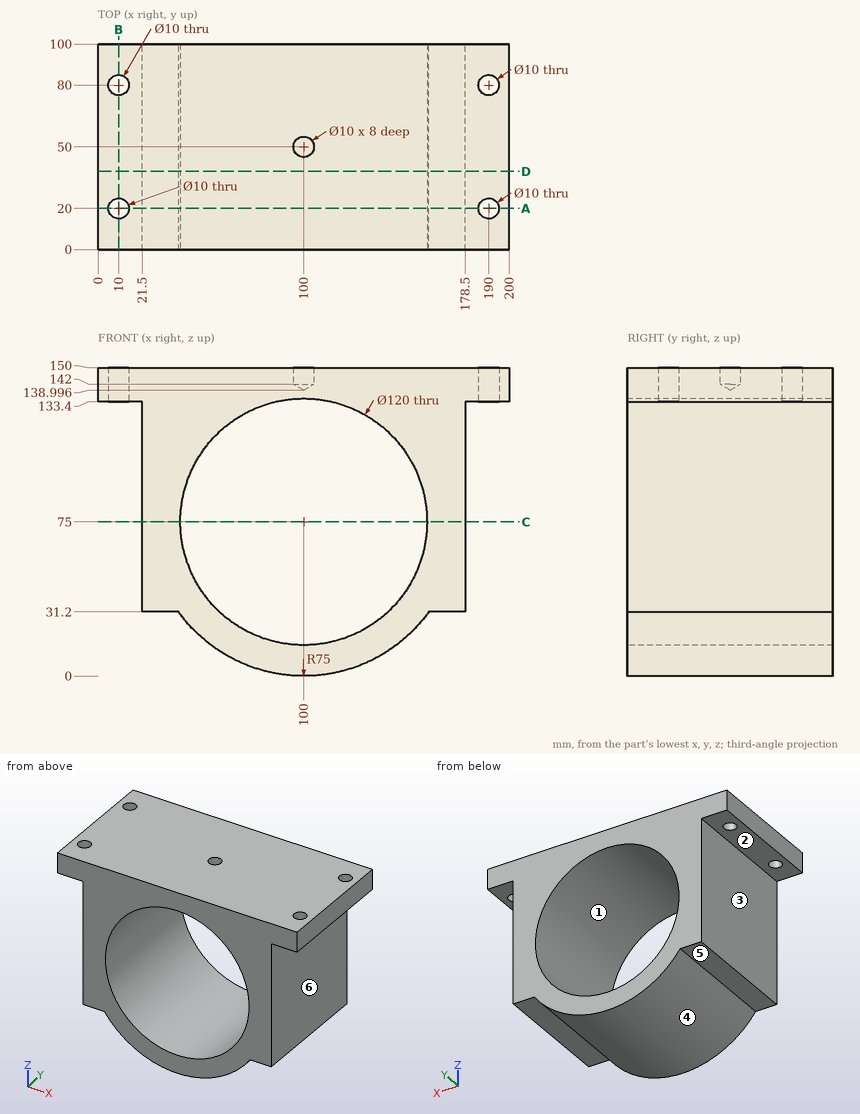
Answer from the drawing. Dimensions are ordinates in mm from the lowest x, y and z of the part. A direction names the side the tool comes from. Give positions to 0.01 mm unless a question says otherwise; leave off trailing zeros. Order: outer loops, then holes, each group sorted by start corner. A loop starts at its lowest first (then second) coordinate and runs counter-clockwise, first axis right, second up. Notation, with made-up numbers: (2.5, 77) - (34.5, 77) arc R22 ccw to (34.5, 100) - close; hole circle Ø10 at (32, 26.5). An arc over 180 degrees is marked (long way). One line per item, written item: value. Start each with the question number.
1) A cutting plane is placed at C-C on z = 75. Give the vertices of the cut face in (x, y), then the cut area to 3 significant figures.
2) A tool of negligible diameter and unlimited length cuts with its end or side. For the marked faces 4, 5 and 6, from which of +Z, -Z, +X, -X, +Y, -Y can it reach the whole face along a straight path? Write none if from no direction.
3) Find the intervals of material crossed by L1, parallel to Y at x = 10, z = 144.5; L2, parallel to Z at x = 98.5, y = 14 (1 decimal); L3, parallel to X at y = 26.5, z = 75, in increasing order.
4) A cutting plane is placed at D-D on y = 38. Give the vertices of the cut face in (x, z).
5) The mould has two halves that part along X. Classify the marked faces 1, 2 and 3: released by +X, released by -X, zero draft, split by the parting line, or undercut.
6) Given pin 1 Ø19.5 at (x, y) = (28.5, 59) entering from -Z; pin 2 Ø8 at (x, y) = (10, 20) entering from -Z; pin 3 Ø16 at (x, y) = (10, 80) entering from -Z; pin 4 Ø3 at (y, z) = (81.5, 27.5) entering from -X, each flat-ended and moving along its own axis, determine where each tip first touches the part or whether it passes through.
7) A cutting plane is placed at A-A on y = 20. Give the vertices of the cut face in (x, z), then the cut area to 3 significant figures.
8) A cutting plane is placed at B-B on x = 10. Give the vertices of the cut face in (y, z).
Answer sheet:
1. outline: (21.5, 0) - (40, 0) - (40, 100) - (21.5, 100) - close; (160, 0) - (178.5, 0) - (178.5, 100) - (160, 100) - close
1. area: 3,700 mm2
2. face 4: -Z, +Y, -Y
2. face 5: -Z, -X, +Y, -Y
2. face 6: -Z, +X, +Y, -Y
3. L1: y = 0 to 15, 25 to 75, 85 to 100
3. L2: z = 0 to 15, 135 to 150
3. L3: x = 21.5 to 40, 160 to 178.5
4. outline: (0, 133.4) - (21.5, 133.4) - (21.5, 31.2) - (39.12, 31.2) arc R75 ccw to (160.88, 31.2) - (178.5, 31.2) - (178.5, 133.4) - (200, 133.4) - (200, 150) - (0, 150) - close; hole circle Ø120 at (100, 75)
5. face 1: undercut
5. face 2: zero draft
5. face 3: released by -X
6. pin 1: stops at z = 31.2
6. pin 2: passes through
6. pin 3: stops at z = 133.4
6. pin 4: stops at x = 40.76
7. outline: (0, 133.4) - (5, 133.4) - (5, 150) - (0, 150) - close; (15, 133.4) - (21.5, 133.4) - (21.5, 31.2) - (39.12, 31.2) arc R75 ccw to (160.88, 31.2) - (178.5, 31.2) - (178.5, 133.4) - (185, 133.4) - (185, 150) - (15, 150) - close; (195, 133.4) - (200, 133.4) - (200, 150) - (195, 150) - close; hole circle Ø120 at (100, 75)
7. area: 10,400 mm2
8. outline: (0, 133.4) - (15, 133.4) - (15, 150) - (0, 150) - close; (25, 133.4) - (75, 133.4) - (75, 150) - (25, 150) - close; (85, 133.4) - (100, 133.4) - (100, 150) - (85, 150) - close
